Drawing for the job (mm, zero at the part's lowest x, y, z). A direction names the side the tool comes from. Round coordinates to 2 decimals unless told otherwise and drop trailing zeros. Order: outer loops, then holes, each group sorted by start corner. A loop starts at its lowest first (then second) coordinate and runs counter-clockwise, first axis right, second up. Notation, with made-up numbers: (39, 9) - (78, 9) arc R24 cw to (78, 22) - close; hole circle Ø1 at (29.25, -5.75). An arc over 180 degrees is marked (long way). Answer as a JSON object with one key per item and string values.
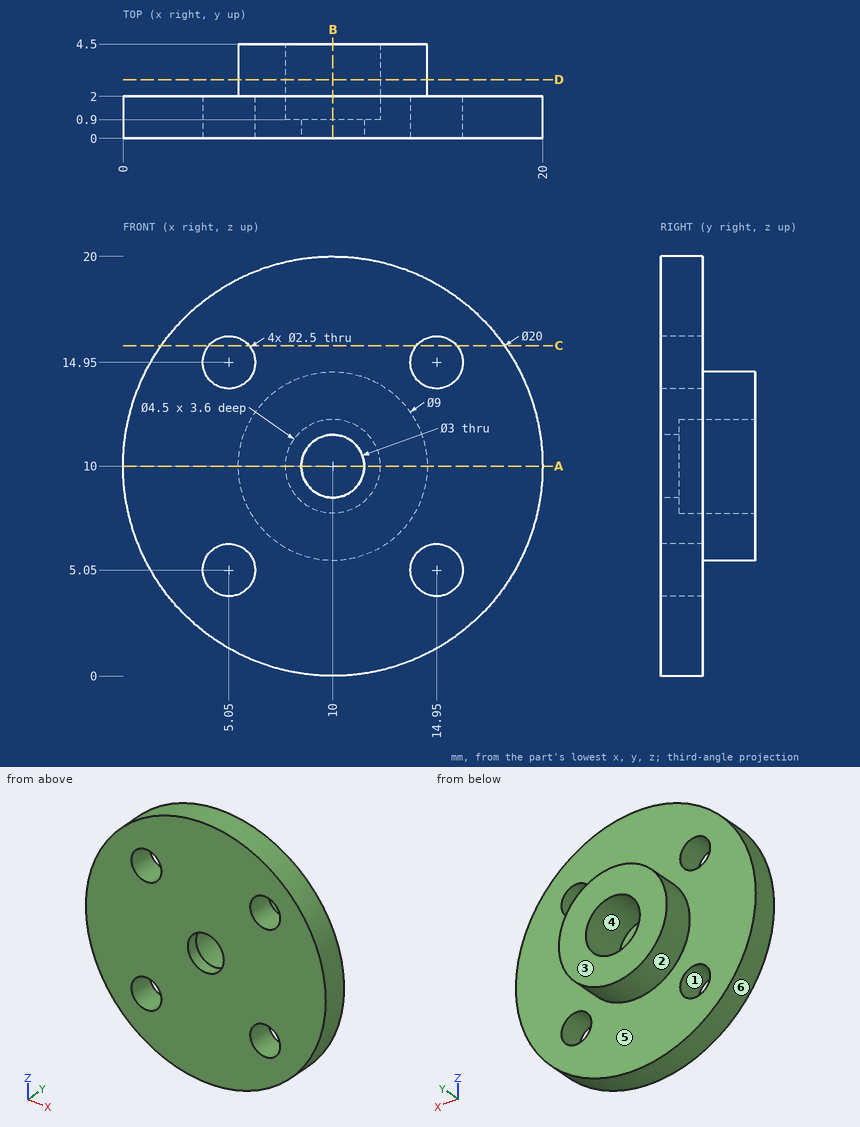
Item 1: Drop flat-ended pins along their axis: P1, Ø4, axis at x = 5, z = 4.5, coming from the +Y side; P2, Ø2, axis at x = 10.5, z = 11, coming from the +Y side; P3, Ø2, axis at x = 11.5, y = 2, coming from the +Z side. Give the stop position or say it passes through.
Taken from the geometry:
{"P1": "y = 2", "P2": "y = 0.9", "P3": "z = 19.99"}
Item 2: Two-plate mould, pull along Z, no slides. Class the marked faces 1, 2, 3 and 4: pulls with the +Z half, pulls with the -Z half, needs draft (parallel to the pull), parting line crosses it, or undercut.
Taken from the geometry:
{"face 1": "undercut", "face 2": "parting line crosses it", "face 3": "needs draft", "face 4": "undercut"}
Item 3: Probe L1, parallel to Z at x = 10, y = 0.65; L2, parallel to Z at x = 10, y = 1.8; L3, parallel to X at y = 0.95, z = 4.5. List the from-to ranges inside material, lowest first. Write a range as from..to.
Taken from the geometry:
{"L1": "0..8.5, 11.5..20", "L2": "0..7.75, 12.25..20", "L3": "1.65..3.93, 6.17..13.83, 16.07..18.35"}
Item 4: Cut at D-D (y = 2.8). Write the cut outline in (x, z).
Taken from the geometry:
{"outline": "circle Ø9 at (10, 10); hole circle Ø4.5 at (10, 10)"}
Item 5: Cut at C-C (z = 15.75). Write the cut outline in (x, y).
Taken from the geometry:
{"outline": "(1.82, 0) - (4.09, 0) - (4.09, 2) - (1.82, 2) - close; (6.01, 0) - (13.99, 0) - (13.99, 2) - (6.01, 2) - close; (15.91, 0) - (18.18, 0) - (18.18, 2) - (15.91, 2) - close"}
Item 6: Tool access for the marked faces 5 and 6: list every direction of +Z, -Z, +X, -X, +Y, -Y with a clear straight run to the whole face (end or side of a thin tool).
Taken from the geometry:
{"face 5": "+Y", "face 6": "+Y, -Y"}
Item 7: Cut at A-A (z = 10). Write the cut outline in (x, y), plus the area to 3 significant figures.
Taken from the geometry:
{"outline": "(0, 0) - (8.5, 0) - (8.5, 0.9) - (7.75, 0.9) - (7.75, 4.5) - (5.5, 4.5) - (5.5, 2) - (0, 2) - close; (11.5, 0) - (20, 0) - (20, 2) - (14.5, 2) - (14.5, 4.5) - (12.25, 4.5) - (12.25, 0.9) - (11.5, 0.9) - close", "area": "43.6 mm2"}
Item 8: Cut at B-B (x = 10). Write the cut outline in (y, z), plus the area to 3 significant figures.
Taken from the geometry:
{"outline": "(0, 0) - (2, 0) - (2, 5.5) - (4.5, 5.5) - (4.5, 7.75) - (0.9, 7.75) - (0.9, 8.5) - (0, 8.5) - close; (0, 11.5) - (0.9, 11.5) - (0.9, 12.25) - (4.5, 12.25) - (4.5, 14.5) - (2, 14.5) - (2, 20) - (0, 20) - close", "area": "43.6 mm2"}
